Can you work these out from the model? Positions are in its coordinate system, mm. A direction names the side the tool comes from. Give positions to 0.01 mm unless a question says otherwise; leave off trailing zeros. Order: outer loops, then holes, each group sorted by start corner. A loop starts at its lowest first (then second) coordinate and runs counter-clockwise, first axis right, second up. Notation, with made-up numbers: (17, -23.75) - (40, -23.75) arc R13 ccw to (40, -2.75) - close; hole circle Ø5 at (25.25, 46). An arc over 180 degrees is marked (long way). Return JSON: item names as keys, results as strings.
```python
from build123d import *

# Parameters (mm, degrees)
SKETCH1_W           = 150
SKETCH1_H           = 250
BOSS_EXTRUDE1_DEPTH = 25
SKETCH2_W           = 134
SKETCH2_H           = 234
CUT_EXTRUDE1_DEPTH  = 51
CUT_EXTRUDE2_DEPTH  = 251
SKETCH7_W           = 1.5
SKETCH7_H           = 2
CUT_EXTRUDE5_DEPTH  = 49
FILLET1_R           = 5
FILLET2_R           = 3
FILLET3_R           = 0.3


with BuildPart() as part:
    # Sketch1 → Boss-Extrude1 (new body, symmetric)
    with BuildSketch(Plane.XY):
        with Locations((75, 125)):
            Rectangle(SKETCH1_W, SKETCH1_H)
    extrude(amount=BOSS_EXTRUDE1_DEPTH, both=True)

    # Sketch2 → Cut-Extrude1 (cut, through all)
    with BuildSketch(Plane.XY.offset(25)):
        with Locations((75, 125)):
            Rectangle(SKETCH2_W, SKETCH2_H)
    extrude(amount=-CUT_EXTRUDE1_DEPTH, mode=Mode.SUBTRACT)

    # Sketch3 → Cut-Extrude2 (cut, through all)
    with BuildSketch(Plane(origin=(0, 250, 0), x_dir=(1, 0, 0), z_dir=(0, 1, 0))):
        with BuildLine():
            Line((73.09, -1.836954001), (76.91, -1.836954001))
            ThreePointArc((76.91, -1.836954001), (75, 2.65), (73.09, -1.836954001))
        make_face()
    extrude(amount=-CUT_EXTRUDE2_DEPTH, mode=Mode.SUBTRACT)

    # Sketch7 → Cut-Extrude5 (cut)
    with BuildSketch(Plane.XY.offset(25)):
        with Locations((7.25, 181)):
            Rectangle(SKETCH7_W, SKETCH7_H)
        with Locations((7.25, 228)):
            Rectangle(SKETCH7_W, SKETCH7_H)
        with Locations((7.25, 170)):
            Rectangle(SKETCH7_W, SKETCH7_H)
        with Locations((7.25, 80)):
            Rectangle(SKETCH7_W, SKETCH7_H)
        with Locations((7.25, 22)):
            Rectangle(SKETCH7_W, SKETCH7_H)
        with Locations((7.25, 69)):
            Rectangle(SKETCH7_W, SKETCH7_H)
        with Locations((7.25, 130.5)):
            Rectangle(SKETCH7_W, SKETCH7_H)
        with Locations((7.25, 119.5)):
            Rectangle(SKETCH7_W, SKETCH7_H)
        with Locations((142.75, 119.5)):
            Rectangle(SKETCH7_W, SKETCH7_H)
        with Locations((142.75, 130.5)):
            Rectangle(SKETCH7_W, SKETCH7_H)
        with Locations((142.75, 69)):
            Rectangle(SKETCH7_W, SKETCH7_H)
        with Locations((142.75, 22)):
            Rectangle(SKETCH7_W, SKETCH7_H)
        with Locations((142.75, 80)):
            Rectangle(SKETCH7_W, SKETCH7_H)
        with Locations((142.75, 170)):
            Rectangle(SKETCH7_W, SKETCH7_H)
        with Locations((142.75, 181)):
            Rectangle(SKETCH7_W, SKETCH7_H)
        with Locations((142.75, 228)):
            Rectangle(SKETCH7_W, SKETCH7_H)
    extrude(amount=-CUT_EXTRUDE5_DEPTH, mode=Mode.SUBTRACT)

    # Fillet1
    fillet1_edges = [part.edges().sort_by_distance(p)[0] for p in [
        (142, 242, 0),
        (142, 8, 0),
        (8, 8, 0),
        (8, 242, 0),
        (0, 250, 0),
        (150, 250, 0),
        (150, 0, 0),
        (0, 0, 0),
    ]]
    fillet(fillet1_edges, radius=FILLET1_R)

    # Fillet2
    fillet2_edges = [part.edges().sort_by_distance(p)[0] for p in [
        (150, 125, -25),
        (150, 125, 25),
        (0, 125, -25),
        (75, 250, -25),
        (75, 0, -25),
        (1.464466094, 248.535533906, -25),
        (148.535533906, 248.535533906, -25),
        (1.464466094, 1.464466094, -25),
        (148.535533906, 1.464466094, -25),
        (75, 0, 25),
        (0, 125, 25),
        (75, 250, 25),
        (1.464466094, 248.535533906, 25),
        (148.535533906, 248.535533906, 25),
        (1.464466094, 1.464466094, 25),
        (148.535533906, 1.464466094, 25),
    ]]
    fillet(fillet2_edges, radius=FILLET2_R)

    # Fillet3
    fillet3_edges = [part.edges().sort_by_distance(p)[0] for p in [
        (6.5, 70, 0.5),
        (8, 70, 0.5),
        (6.5, 129.5, 0.5),
        (6.5, 131.5, 0.5),
        (8, 131.5, 0.5),
        (8, 129.5, 0.5),
        (6.5, 118.5, 0.5),
        (6.5, 120.5, 0.5),
        (8, 120.5, 0.5),
        (8, 118.5, 0.5),
        (143.5, 131.5, 0.5),
        (143.5, 129.5, 0.5),
        (142, 129.5, 0.5),
        (142, 131.5, 0.5),
        (8, 21, 0.5),
        (6.5, 21, 0.5),
        (6.5, 23, 0.5),
        (8, 23, 0.5),
        (6.5, 79, 0.5),
        (6.5, 81, 0.5),
        (8, 81, 0.5),
        (8, 79, 0.5),
        (6.5, 169, 0.5),
        (6.5, 171, 0.5),
        (8, 171, 0.5),
        (8, 169, 0.5),
        (6.5, 227, 0.5),
        (6.5, 229, 0.5),
        (8, 229, 0.5),
        (8, 227, 0.5),
        (143.5, 81, 0.5),
        (143.5, 79, 0.5),
        (142, 79, 0.5),
        (142, 81, 0.5),
        (143.5, 23, 0.5),
        (143.5, 21, 0.5),
        (142, 21, 0.5),
        (142, 23, 0.5),
        (143.5, 70, 0.5),
        (143.5, 68, 0.5),
        (142, 68, 0.5),
        (142, 70, 0.5),
        (142, 120.5, 0.5),
        (143.5, 120.5, 0.5),
        (143.5, 118.5, 0.5),
        (142, 118.5, 0.5),
        (142, 171, 0.5),
        (143.5, 171, 0.5),
        (143.5, 169, 0.5),
        (142, 169, 0.5),
        (142, 182, 0.5),
        (143.5, 182, 0.5),
        (143.5, 180, 0.5),
        (142, 180, 0.5),
        (142, 229, 0.5),
        (143.5, 229, 0.5),
        (143.5, 227, 0.5),
        (142, 227, 0.5),
        (6.5, 180, 0.5),
        (6.5, 182, 0.5),
        (8, 182, 0.5),
        (8, 180, 0.5),
        (8, 68, 0.5),
        (6.5, 68, 0.5),
    ]]
    fillet(fillet3_edges, radius=FILLET3_R)


solid = part.part
```
1. Thinking about a two-plate mould opening in X: for faces 1 (the face through (1, 248, 0)), 2 (the face through (142, 123, 0)), 3 (the face through (150, 123, 0)), 4 (the face through (10, 9, 0)), which applies, +X half, -X half, draft (parallel to the pull), parting line (faces both ways), or undercut?
Checks:
{"face 1": "-X half", "face 2": "undercut", "face 3": "+X half", "face 4": "undercut"}
2. On a 3-axis mill with a long thin cutter (end or side, diameter ignored), from which of +Z, -Z, +X, -X, +Y, -Y can I reach the whole of each face in a straight line? I mean faces 5 (the face through (148, 249, 0)), 6 (the face through (74, 8, 6)). Say none if no direction works.
Checks:
{"face 5": "+Z, -Z, +X, +Y", "face 6": "+Z, -Z"}
3. Suppose I cut it at A-A (y = 114.5). List the corners of the cut face in (x, z) for me.
Checks:
{"outline": "(0, -22) arc R3 ccw to (3, -25) - (8, -25) - (8, 25) - (3, 25) arc R3 ccw to (0, 22) - close; (142, -25) - (147, -25) arc R3 ccw to (150, -22) - (150, 22) arc R3 ccw to (147, 25) - (142, 25) - close"}
4. Suppose I cut it at B-B (x = 84). List the corners of the cut face in (y, z) for me, plus the area to 3 significant figures.
Checks:
{"outline": "(0, -22) arc R3 ccw to (3, -25) - (8, -25) - (8, 25) - (3, 25) arc R3 ccw to (0, 22) - close; (242, -25) - (247, -25) arc R3 ccw to (250, -22) - (250, 22) arc R3 ccw to (247, 25) - (242, 25) - close", "area": "792 mm^2"}
5. If I drill on L1, parallel to X at y = 36.5, z = -8; L2, parallel to Y at x = 23, z = -9; L3, parallel to Z at x = 75, y = 6.25, over which ranges is the centre line in solid material (lowest first)? Write a range as [from, to].
Checks:
{"L1": "[0, 8], [142, 150]", "L2": "[0, 8], [242, 250]", "L3": "[-25, -2.65], [1.84, 25]"}
6. For pin 1 Ø0.8 at (x, y) = (7, 80) entering from +Z, with a flat end and sliding along its axis, tell me the tip position at first contact or that it passes through.
Checks:
{"pin 1": "z = -24"}
